Read the model definition and answer for the solid it produces. Units are mm, in the model's axes. A direction names the side the tool comes from. Coordinates: 2 decimals unless noted, no trailing zeros. Write each loop counter-clockwise with the first axis right and the second up, starting at its lowest first coordinate (ties: lowest second). Pieces come first, ordered by that corner, then holes. Notation, with made-up numbers: (80, 20.25) -> (129, 20.25) arc R12 ccw to (129, 24.25) -> close; hole circle Ø10 at (71, 56.25). An arc over 180 degrees is marked (long way). Return JSON: item names as keys, results as strings.
from build123d import *

# Parameters (mm, degrees)
F2_DEPTH      = 80
F2_DEPTH_BACK = 80
F3_START      = -34.501
F3_DEPTH      = 119.002


with BuildPart() as f2:
    # F0 (on Front) → F2 (new body, two sides)
    with BuildSketch(Plane.XZ) as f2_sk:
        with BuildLine():
            Line((25, 115), (25, 110))
            Line((25, 110), (74.5, 110))
            ThreePointArc((74.5, 110), (78.0355339059, 108.5355339059), (79.5, 105))
            Line((79.5, 105), (79.5, 0))
            Line((79.5, 0), (79.5, -20))
            Line((79.5, -20), (84.5, -20))
            Line((84.5, -20), (84.5, 105))
            ThreePointArc((84.5, 105), (81.5710678119, 112.0710678119), (74.5, 115))
            Line((74.5, 115), (25, 115))
        make_face()
        with BuildLine():
            Line((-29.5, -20), (-29.5, 0))
            Line((-29.5, 0), (-29.5, 105))
            ThreePointArc((-29.5, 105), (-28.0355339059, 108.5355339059), (-24.5, 110))
            Line((-24.5, 110), (25, 110))
            Line((25, 110), (25, 115))
            Line((25, 115), (-24.5, 115))
            ThreePointArc((-24.5, 115), (-31.5710678119, 112.0710678119), (-34.5, 105))
            Line((-34.5, 105), (-34.5, -20))
            Line((-34.5, -20), (-29.5, -20))
        make_face()
    extrude(amount=F2_DEPTH)
    extrude(f2_sk.sketch, amount=-F2_DEPTH_BACK)

    # F1 (on Right) → F3 (intersect)
    with BuildSketch(Plane.YZ.offset(F3_START)):
        with BuildLine():
            Line((-60, 115), (-18.9460998047, -6.4066607677))
            ThreePointArc((-18.9460998047, -6.4066607677), (-11.6590476594, -16.2501263896), (0, -20))
            Line((0, -20), (0, -5))
            ThreePointArc((0, -5), (-5, 0), (0, 5))
            Line((0, 5), (0, 115))
            Line((0, 115), (-60, 115))
        make_face()
        with BuildLine():
            Line((0, -5), (0, -20))
            ThreePointArc((0, -20), (11.6590476594, -16.2501263896), (18.9460998047, -6.4066607677))
            Line((18.9460998047, -6.4066607677), (60, 115))
            Line((60, 115), (0, 115))
            Line((0, 115), (0, 5))
            ThreePointArc((0, 5), (3.5355339059, 3.5355339059), (5, 0))
            ThreePointArc((5, 0), (3.5355339059, -3.5355339059), (0, -5))
        make_face()
    extrude(amount=F3_DEPTH, mode=Mode.INTERSECT)


solid = f2.part
1. The part is cut by section B-B (z = 58). Determine the outline of the cut face in (x, y), then the cut area to 3 significant figures.
Taken from the geometry:
{"outline": "(-34.5, -40.73) -> (-29.5, -40.73) -> (-29.5, 40.73) -> (-34.5, 40.73) -> close; (79.5, -40.73) -> (84.5, -40.73) -> (84.5, 40.73) -> (79.5, 40.73) -> close", "area": "815 mm2"}
2. Flat-ended cylindrical pins translate along their axes: pin 1 Ø5 at (x, y) = (-3.5, -32.5) entering from -Z; pin 2 Ø3 at (y, z) = (34, 36) entering from -X. Find the tip coordinate at first contact, or state that the pin passes through.
Taken from the geometry:
{"pin 1": "stops at z = 110", "pin 2": "stops at x = -34.5"}
3. A tool of negligible diameter and unlimited length cuts with its end or side. For faces 4 (the face through (24, -1, 110)), 5 (the face through (-34.5, -1, 57)), from which of +Z, -Z, +X, -X, +Y, -Y can it reach the whole face along a straight path? Write none if from no direction.
Taken from the geometry:
{"face 4": "-Z, +Y, -Y", "face 5": "+Z, -Z, -X, +Y, -Y"}
4. Consider L1, parallel to X at y = 38, z = 89.5; L2, parallel to Z at x = 0, y = 19; L3, parallel to X at y = -6.5, z = 108. Determine where each line is inside the solid, lowest interval first.
Taken from the geometry:
{"L1": "x = -34.5 to -29.5, 79.5 to 84.5", "L2": "z = 110 to 115", "L3": "x = -34.04 to -28.5, 78.5 to 84.04"}
5. For a pull along X with two mould halves and no side action, classify faces 1 (the face through (-31.49, -0.84, 112.15)), 2 (the face through (24.722, -59.336, 113.035)), 3 (the face through (-28.07, -0.82, 108.5)) as +X half, -X half, draft (parallel to the pull), parting line (faces both ways), or undercut.
Taken from the geometry:
{"face 1": "-X half", "face 2": "draft", "face 3": "undercut"}
6. The part is cut by section C-C (x = 59.5). Determine the outline of the cut face in (y, z).
Taken from the geometry:
{"outline": "(-60, 115) -> (-58.31, 110) -> (58.31, 110) -> (60, 115) -> close"}
7. The part is cut by section A-A (z = 26). Determine the outline of the cut face in (x, y), then the cut area to 3 significant figures.
Taken from the geometry:
{"outline": "(-34.5, -29.9) -> (-29.5, -29.9) -> (-29.5, 29.9) -> (-34.5, 29.9) -> close; (79.5, -29.9) -> (84.5, -29.9) -> (84.5, 29.9) -> (79.5, 29.9) -> close", "area": "598 mm2"}
